Answer from the drawing. Dimensions are ordinates in mm from the lowest x, y and z of the part. A direction names the side the tool comes from. Coordinates: 2 decimals unless noted, no trailing zeros. Write each loop counter-clockwise with the first axis right and the second up, starting at its lowest first coordinate (ties: lowest second). Pieces come first, ordered by that corner, then holes.
(1) Given P1, Ø3.5, axis at x = 15, y = 11.5, coming from the -Z side; P2, Ø1.5, axis at x = 14.5, y = 7.5, coming from the +Z side; P3, Ø4, axis at y = 10.5, z = 3.5, coming from the +X side; P4, Ø1, axis at y = 9.5, z = 13, coming from the -X side, each flat-ended and moving along its own axis, determine where each tip first touches the part or whether it passes through.
(2) The part is cut by section A-A on z = 2.5. Determine the outline of the cut face in (x, y).
(3) Straight lines are drawn through the part: line 1 (X direction, y = 12, z = 3.5); line 2 (Z direction, x = 21.75, y = 13); line 3 (Z direction, x = 15.5, y = 14). For each, find the intervals that lie inside material, in ascending order.
(4) Which of the six approach directions +Z, -Z, +X, -X, +Y, -Y give full straight-line access (tool end or side, diameter ignored) to the marked faces 5, 6, 7 and 8?
(5) The part is cut by section C-C on y = 13. Determine the outline of the cut face in (x, z).
(6) The part is cut by section B-B on x = 7. Determine the outline of the cut face in (y, z), plus the area to 3 significant figures.
(7) For a pull along X with two mould halves and no side action, classify the marked faces 1, 2, 3 and 4 as +X half, -X half, draft (parallel to the pull), parting line (faces both ways), or undercut.
(8) The part is cut by section D-D on x = 16.25. Determine the outline of the cut face in (y, z).
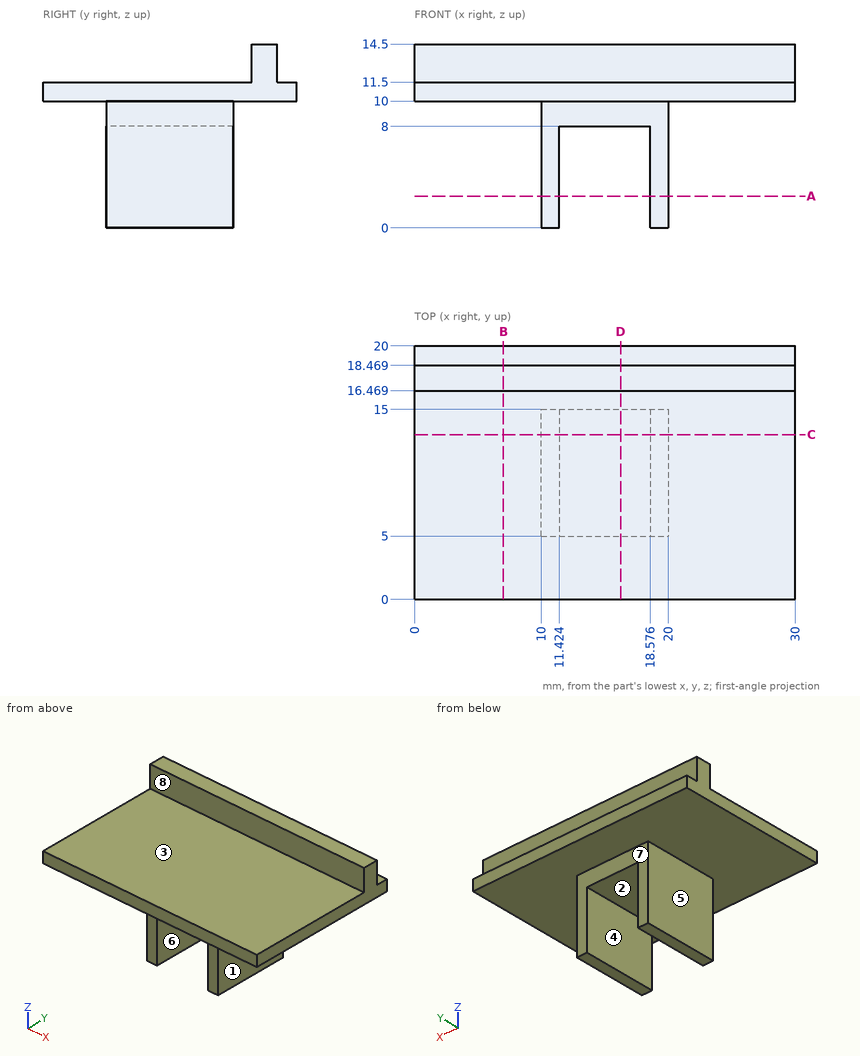
Model answer:
1. P1: stops at z = 8
1. P2: stops at z = 11.5
1. P3: stops at x = 20
1. P4: passes through
2. outline: (10, 5) - (11.42, 5) - (11.42, 15) - (10, 15) - close; (18.58, 5) - (20, 5) - (20, 15) - (18.58, 15) - close
3. line 1: x = 10 to 11.42, 18.58 to 20
3. line 2: z = 10 to 11.5
3. line 3: z = 8 to 11.5
4. face 5: -Z, -X, +Y, -Y
4. face 6: -Z, +Y, -Y
4. face 7: -Z, +X, -X, +Y
4. face 8: +Z, +X, -X, -Y
5. outline: (0, 10) - (10, 10) - (10, 0) - (11.42, 0) - (11.42, 8) - (18.58, 8) - (18.58, 0) - (20, 0) - (20, 10) - (30, 10) - (30, 11.5) - (0, 11.5) - close
6. outline: (0, 10) - (20, 10) - (20, 11.5) - (18.47, 11.5) - (18.47, 14.5) - (16.47, 14.5) - (16.47, 11.5) - (0, 11.5) - close
6. area: 36.0 mm2
7. face 1: +X half
7. face 2: undercut
7. face 3: draft
7. face 4: undercut
8. outline: (0, 10) - (5, 10) - (5, 8) - (15, 8) - (15, 10) - (20, 10) - (20, 11.5) - (18.47, 11.5) - (18.47, 14.5) - (16.47, 14.5) - (16.47, 11.5) - (0, 11.5) - close
